Verification items for this drawing (mm, ordinates from the low corner). A direction names the side the tool comes from. Coordinates: 2 decimals unless noted, no trailing zeros. Write each loop counter-clockwise with the first axis right and the second up, starting at its lowest first coordinate (ties: lowest second). Pieces come first, ordered by that corner, then holes. Notation, with made-up numbers: M 65.25,-8 L 115.25,-8 A21 ccw 115.25,22 Z; hole C -35,40 d10. An arc over 180 degrees is marked long. Write each question's results on one line, items separated by ' | '.
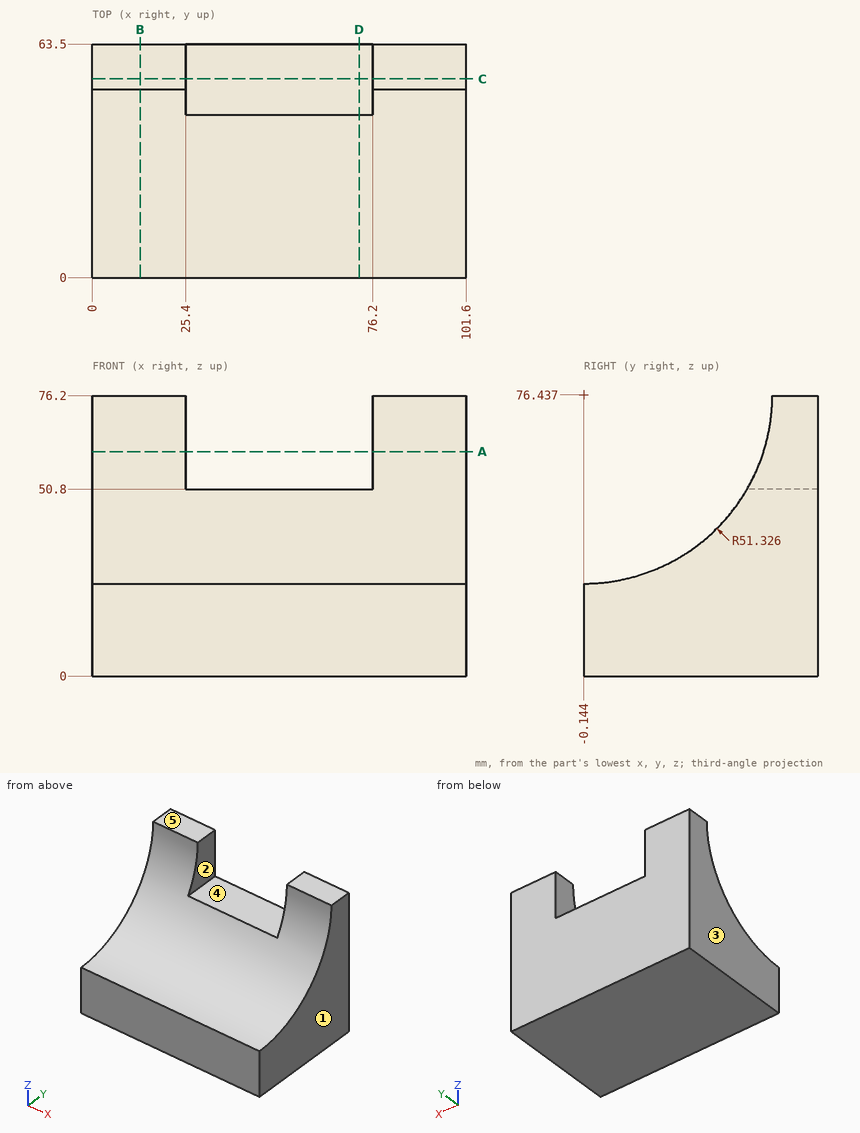
Q1. Access from +Z, -Z, +X, -X, +Y, -Y to the whole of each face (thin tool, end or side, straight path). Record for the marked faces 1 and 2.
Geometry check:
face 1: +Z, -Z, +X, +Y, -Y | face 2: +Z, +Y, -Y
Q2. Sectioned sample at D-D on x = 72.5. Record the cut outline in (y, z) (1 decimal), and give its area (3 significant figures).
Geometry check:
outline: M 0,0 L 63.5,0 L 63.5,50.8 L 44.3,50.8 A51.3 cw 0,25.1 Z | area: 2,420 mm2
Q3. Mould release check, pull along X, two halves, no side actions. Record for the marked faces 3, 4 and 5: pulls with the +X half, pulls with the -X half, needs draft (parallel to the pull), parting line crosses it, or undercut.
Geometry check:
face 3: pulls with the -X half | face 4: undercut | face 5: needs draft
Q4. Sectioned sample at B-B on x = 13. Record the cut outline in (y, z) (1 decimal), and give its area (3 significant figures).
Geometry check:
outline: M 0,0 L 63.5,0 L 63.5,76.2 L 51.2,76.2 A51.3 cw 0,25.1 Z | area: 2,790 mm2
Q5. Sectioned sample at A-A on z = 61. Record the cut outline in (x, y) (1 decimal).
Geometry check:
outline: M 0,48.8 L 25.4,48.8 L 25.4,63.5 L 0,63.5 Z; M 76.2,48.8 L 101.6,48.8 L 101.6,63.5 L 76.2,63.5 Z
Q6. Depth check by flat-ended pin: P1, Ø6, axis at x = 54, y = 50.5, coming from the +Z side; P2, Ø8, axis at x = 53.5, y = 16, coming from the -Z side; P3, Ø10, axis at x = 89.5, y = 38, coming from the +Z side (1 decimal); P4, Ø1, axis at x = 76.5, z = 33, coming from the -Y side (1 decimal). Enter the tip coordinate at first touch or a pass-through.
Geometry check:
P1: stops at z = 50.8 | P2: stops at z = 0 | P3: stops at z = 48.6 | P4: stops at y = 26.4
Q7. Sectioned sample at C-C on y = 54. Record the cut outline in (x, z).
Geometry check:
outline: M 0,0 L 101.6,0 L 101.6,76.2 L 76.2,76.2 L 76.2,50.8 L 25.4,50.8 L 25.4,76.2 L 0,76.2 Z
Q8. Scan lines: probe 1 along X at (y, z) = (54, 60.5); probe 2 along Z at (x, y) = (67, 61); probe 3 along Y at (x, z) = (5, 53). Record each from-to range of solid material in increasing order.
Geometry check:
probe 1: x = 0 to 25.4, 76.2 to 101.6 | probe 2: z = 0 to 50.8 | probe 3: y = 45.52 to 63.5
